Build history of the part. All positions in model axes, mm. A direction names the side the tool comes from. Give positions to 0.01 mm unless a question says otherwise; leave off trailing zeros. Order: outer loops, then holes, each group sorted by start corner. A loop starts at its lowest first (then second) coordinate and runs counter-clockwise, first axis right, second up. Notation, with made-up numbers: (-27.5, 16.5) - (4.5, 16.5) arc R6 ccw to (4.5, 25.5) - close; hole circle Ø7 at (-34.75, 38). An arc over 180 degrees is marked (long way). Use a Markdown table: item, result. Add a question column.
(1) Slice it at C-C (y = 0). Write the cut outline in (x, z), then the cut area to 3 significant figures.
(2) Wall check: line 1 (X direction, y = 3.2, z = -16.51); line 2 (Y direction, x = 8.5, z = -0.5); line 3 (Z direction, x = 15.5, y = -0.25). Give the ranges that are in metal, low to high.
(3) Slice it at B-B (x = 0). Write the cut outline in (y, z).
(4) Slice it at D-D (z = -3.5). Write the cut outline in (x, y), then the cut area to 3 significant figures.
(5) Which spindle directions (+Z, -Z, +X, -X, +Y, -Y) get a long thin tool onto all of the face, cutting with end or side? Do faces 5 (the face through (0, 0, 0)), 6 (the face through (-30.064, -0.594, 0.74)). Say none if no direction does.
(6) Flat gauge pin, fed straight in: pin 1 (8 mm diameter, centred on x = -16.5, z = -21, fed in from -Y). Where does the tip first touch, or does it go through?
(7) Slice it at A-A (z = -16.51). Write the cut outline in (x, y), then the cut area to 3 significant figures.
(8) Mould opens along Y. For faces 1 (the face through (29.947, 0.068, 0.74)), 2 (the face through (-7, 3.532, -16)), 3 (the face through (0, 2.032, -9)), 4 (the face through (34.29, 3, -14)) say: +Y half, -Y half, draft (parallel to the pull), parting line (faces both ways), or undercut.
from build123d import *

# Parameters (mm, degrees)
SKETCH_1_W          = 68.58
SKETCH_1_H          = 4.064
SKETCH_1_R          = 1.55
EXTRUDE_2_DEPTH     = 1.5
SKETCH_3_W          = 68.58
SKETCH_3_H          = 1.5
EXTRUDE_3_DEPTH     = 1.5
SKETCH_4_W          = 68.58
SKETCH_4_H          = 1.5
EXTRUDE_4_DEPTH     = 33.02
SKETCH_5_R          = 5.334
CUT_EXTRUDE_2_DEPTH = 33.02


with BuildPart() as part:
    # 草图1 → 凸台-拉伸2 (new body)
    with BuildSketch(Plane.XY):
        Rectangle(SKETCH_1_W, SKETCH_1_H)
        with Locations((31.496, 0)):
            Circle(SKETCH_1_R, mode=Mode.SUBTRACT)
        with Locations((-31.496, 0)):
            Circle(SKETCH_1_R, mode=Mode.SUBTRACT)
    extrude(amount=EXTRUDE_2_DEPTH)

    # 草图3 → 凸台-拉伸3 (add)
    with BuildSketch(Plane(origin=(0, 2.032, 0), x_dir=(1, 0, 0), z_dir=(0, 1, 0))):
        with Locations((0, -0.75)):
            Rectangle(SKETCH_3_W, SKETCH_3_H)
    extrude(amount=EXTRUDE_3_DEPTH)

    # 草图4 → 凸台-拉伸4 (add)
    with BuildSketch(Plane(origin=(0, 0, 0), x_dir=(-1, 0, 0), z_dir=(0, 0, -1))):
        with Locations((0, 2.782)):
            Rectangle(SKETCH_4_W, SKETCH_4_H)
    extrude(amount=EXTRUDE_4_DEPTH)

    # 草图5 → 切除-拉伸2 (cut)
    with BuildSketch(Plane.XZ.offset(-2.032)):
        with Locations(Location((0, -16.51, 0), (0, 0, 270))):
            Circle(SKETCH_5_R)
    extrude(amount=-CUT_EXTRUDE_2_DEPTH, mode=Mode.SUBTRACT)


solid = part.part
Solution:
| question | item | result |
|---|---|---|
| 1 | outline | (-34.29, 0) - (-33.05, 0) - (-33.05, 1.5) - (-34.29, 1.5) - close; (-29.95, 0) - (29.95, 0) - (29.95, 1.5) - (-29.95, 1.5) - close; (33.05, 0) - (34.29, 0) - (34.29, 1.5) - (33.05, 1.5) - close |
| 1 | area | 93.6 mm2 |
| 2 | line 1 | -34.29 to -5.33, 5.33 to 34.29 |
| 2 | line 2 | 2.03 to 3.53 |
| 2 | line 3 | 0 to 1.5 |
| 3 | outline | (-2.03, 0) - (2.03, 0) - (2.03, -11.18) - (3.53, -11.18) - (3.53, 1.5) - (-2.03, 1.5) - close; (2.03, -33.02) - (3.53, -33.02) - (3.53, -21.84) - (2.03, -21.84) - close |
| 4 | outline | (-34.29, 2.03) - (34.29, 2.03) - (34.29, 3.53) - (-34.29, 3.53) - close |
| 4 | area | 103 mm2 |
| 5 | face 5 | -Z, +X, -X, -Y |
| 5 | face 6 | +Z, -Z |
| 6 | pin 1 | y = 2.03 |
| 7 | outline | (-34.29, 2.03) - (-5.33, 2.03) - (-5.33, 3.53) - (-34.29, 3.53) - close; (5.33, 2.03) - (34.29, 2.03) - (34.29, 3.53) - (5.33, 3.53) - close |
| 7 | area | 86.9 mm2 |
| 8 | face 1 | undercut |
| 8 | face 2 | +Y half |
| 8 | face 3 | -Y half |
| 8 | face 4 | draft |
